Could you check a few things on this model? Use its own coordinates, in mm. Face numbers are marked on the shaded views. A direction names the side the tool comes from. Give positions to 0.01 mm unless a question says otherwise; leave off trailing zeros. Order: outer loops, then holes, each group sorted by start corner. A loop starts at its lowest first (then second) coordinate and runs counter-clockwise, first axis right, second up. Notation, with made-up numbers: (3.25, 34.25) -> (56.25, 34.25) arc R29 cw to (56.25, 64.25) -> close; hole circle Ø2 at (33.5, 10). An arc over 180 degrees is marked (long way). Write each question's results on one line, items separated by ' | '.
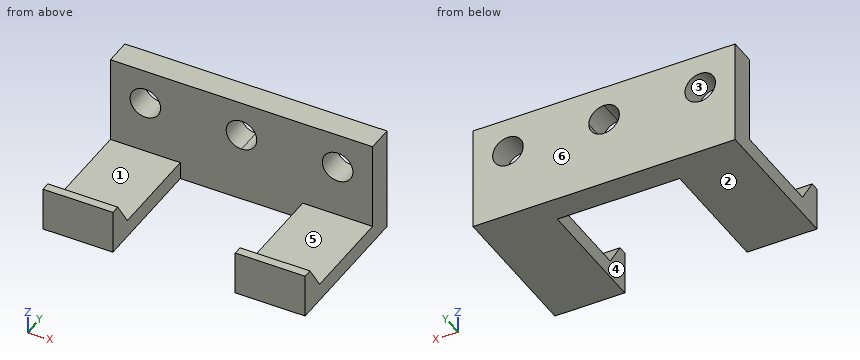
```python
from build123d import *

# Parameters (mm, degrees)
F0_W     = 8
F0_H     = 14
F1_DEPTH = 2
F3_DEPTH = 10
F4_R     = 1.75
F5_DEPTH = 25
F7_DEPTH = 30
F8_W     = 14
F8_H     = 3
F9_DEPTH = 25


with BuildPart() as f1:
    # F0 (on Top) → F1 (new body)
    with BuildSketch(Plane.XY):
        with Locations((-26, -7)):
            Rectangle(F0_W, F0_H)
        Polygon((-22, 0), (-15, 0), (-15, 3), (-30, 3), (-30, 0), align=None)
        Polygon((-8, 0), (0, 0), (0, 3), (-15, 3), (-15, 0), align=None)
        with Locations((-4, -7)):
            Rectangle(F0_W, F0_H)
    extrude(amount=F1_DEPTH)

    # F2 (on face) → F3 (join)
    with BuildSketch(Plane.XY.offset(2)):
        Polygon((0, 3), (-30, 3), (-30, 0), (-22, 0), (-8, 0), (0, 0), align=None)
    extrude(amount=F3_DEPTH)

    # F4 (on face) → F5 (cut)
    with BuildSketch(Plane.XZ):
        with Locations((-26, 8)):
            Circle(F4_R)
        with BuildLine():
            Line((-15, 6.25), (-15, 9.75))
            ThreePointArc((-15, 9.75), (-16.75, 8), (-15, 6.25))
        make_face()
        with BuildLine():
            ThreePointArc((-13.25, 8), (-13.7625631329, 9.2374368671), (-15, 9.75))
            Line((-15, 9.75), (-15, 6.25))
            ThreePointArc((-15, 6.25), (-13.7625631329, 6.7625631329), (-13.25, 8))
        make_face()
        with Locations((-4, 8)):
            Circle(F4_R)
    extrude(amount=-F5_DEPTH, mode=Mode.SUBTRACT)

    # F6 (on face) → F7 (join)
    with BuildSketch(Plane(origin=(-30, 0, 0), x_dir=(0, -1, 0), z_dir=(-1, 0, 0))):
        Polygon((11, 2), (14, 2), (14, 5), (13, 5), align=None)
    extrude(amount=-F7_DEPTH)

    # F8 (on face) → F9 (cut)
    with BuildSketch(Plane(origin=(0, 0, 2), x_dir=(1, 0, 0), z_dir=(0, 0, -1))):
        with Locations((-15, 12.5)):
            Rectangle(F8_W, F8_H)
    extrude(amount=-F9_DEPTH, mode=Mode.SUBTRACT)


solid = f1.part
```
Q1. Suppose I cut it at D-D on z = 1. Please give me the cut outline in (x, y).
Here are the results:
outline: (-30, -14) -> (-22, -14) -> (-22, 0) -> (-8, 0) -> (-8, -14) -> (0, -14) -> (0, 3) -> (-30, 3) -> close
Q2. Suppose I cut it at C-C on z = 7.25. Please give me the cut outline in (x, y), and give its area (3 significant figures).
Here are the results:
outline: (-30, 0) -> (-27.58, 0) -> (-27.58, 3) -> (-30, 3) -> close; (-24.42, 0) -> (-16.58, 0) -> (-16.58, 3) -> (-24.42, 3) -> close; (-13.42, 0) -> (-5.58, 0) -> (-5.58, 3) -> (-13.42, 3) -> close; (-2.42, 0) -> (0, 0) -> (0, 3) -> (-2.42, 3) -> close | area: 61.5 mm²
Q3. I'm going to push flat-ended pins straight in: pin 1 Ø0.5 at (x, y) = (-2, -13.5) entering from +Z; pin 2 Ø2.5 at (x, y) = (-25, -6) entering from +Z; pin 3 Ø6 at (y, z) = (-1.5, 10.5) entering from +X; pin 4 Ø5 at (x, z) = (-18, 9) entering from -Y. Where does each tip first touch, or does it pass through?
Here are the results:
pin 1: stops at z = 5 | pin 2: stops at z = 2 | pin 3: stops at x = 0 | pin 4: stops at y = 0
Q4. Suppose I cut it at B-B on x = -4. Please give me the cut outline in (y, z).
Here are the results:
outline: (-14, 0) -> (3, 0) -> (3, 6.25) -> (0, 6.25) -> (0, 2) -> (-11, 2) -> (-13, 5) -> (-14, 5) -> close; (0, 9.75) -> (3, 9.75) -> (3, 12) -> (0, 12) -> close
Q5. Suppose I cut it at A-A on y = -9.25. Please give me the cut outline in (x, z).
Here are the results:
outline: (-30, 0) -> (-22, 0) -> (-22, 2) -> (-30, 2) -> close; (-8, 0) -> (0, 0) -> (0, 2) -> (-8, 2) -> close
Q6. For the marked faces 4, 5 and 6, which set-ups out of +Z, -Z, +X, -X, +Y, -Y let a thin tool reach every point of the face, with its end or its side?
Here are the results:
face 4: +Z, -Z, -Y | face 5: +Z, +X, -X | face 6: +Z, -Z, +X, -X, +Y
Q7. Thinking about a two-plate mould opening in Z: for the marked faces 1, 2 and 3, which applies, +Z half, -Z half, draft (parallel to the pull), parting line (faces both ways), or undercut?
Here are the results:
face 1: +Z half | face 2: -Z half | face 3: undercut
Q8. I need wall thicknesses on line 1 along Z through (x, y) = (-4, 1); line 2 along Y through (x, z) = (-20.25, 7.75); line 3 along X through (y, z) = (1, 8.75). Which ranges of each line are inside material? Lowest first, please.
Here are the results:
line 1: z = 0 to 6.25, 9.75 to 12 | line 2: y = 0 to 3 | line 3: x = -30 to -27.58, -24.42 to -16.58, -13.42 to -5.58, -2.42 to 0
